Verification items for the finished model (mm, model axes). A direction names the side the tool comes from. Coordinates: 2 decimals unless noted, no trailing zeros. Order: outer loops, then holes, each group sorted by start corner. A loop starts at its lowest first (then second) coordinate and runs counter-clockwise, first axis right, second up. Notation, with made-up numbers: (33, 0.25) -> (63, 0.25) arc R31 ccw to (63, 38.25) -> close; hole circle Ø1 at (-8, 55.5). An arc over 180 degrees is marked (long way). Use CSV: the item, a comma, the result in double quotes. Start each with the question number.
1) Sectioned sample at C-C on z = 0. Record the boundary of the cut face in (x, y).
2) Release check for a two-part mould opening along Z. For faces 1 (the flat face through (0, 6, -30)), 2 (the flat face through (20, 2, -24.207)), 3 (the cylindrical face through (-0.521, 15.966, 28.986)) record: released by +Z, released by -Z, zero draft, split by the parting line, or undercut.
3) Sectioned sample at D-D on y = 12. Record the boundary of the cut face in (x, z).
4) Tool access check on faces 4 (the flat face through (-7, 2, 24)), 5 (the flat face through (0, 6, 30)), 6 (the flat face through (18, 18, -27)). Record the directions out of +Z, -Z, +X, -X, +Y, -Y that give a thin tool (end or side, any length) a straight path to the whole face; none if there is none.
5) Go/stop test with flat-tipped pins: pin 1 (2.5 mm diameter, centred on y = 20.5, z = -22.5, fed in from -X); pin 2 (1.5 mm diameter, centred on y = 9, z = 1.5, fed in from +X); pin 3 (1 mm diameter, centred on x = 18, z = 27.5, fed in from +Y). Record where each tip stops, or that it passes through.
6) Sectioned sample at A-A on y = 5.5. Give the number of separate pieces and of enclosed holes in the cut face, then the cut area to 3 significant figures.
7) Scan lines: line 1 along X through (y, z) = (19.3, -27.5); line 2 along Y through (x, z) = (15.5, -22.5); line 3 along X through (y, z) = (19, 4). Record each from-to range of solid material in increasing order.
8) Sectioned sample at B-B on x = 0. Record the boundary of the cut face in (y, z), then the cut area to 3 significant figures.
from build123d import *

# Parameters (mm, degrees)
CROQUIS2_R                 = 1.5
SALIENTE_EXTRUIR1_DEPTH    = 3
CROQUIS3_W                 = 1.97
CROQUIS3_H                 = 56
SALIENTE_EXTRUIR2_DEPTH    = 20
CROQUIS4_W                 = 4.999751321
CROQUIS4_H                 = 20
SALIENTE_EXTRUIR3_DEPTH    = 5
CROQUIS5_W                 = 5
CROQUIS5_H                 = 20
SALIENTE_EXTRUIR4_DEPTH    = 5
CROQUIS6_R                 = 1
CORTAR_EXTRUIR1_DEPTH      = 5
CROQUIS7_R                 = 1
CORTAR_EXTRUIR2_DEPTH      = 67.738294854
CROQUIS8_R                 = 1
CORTAR_EXTRUIR3_DEPTH      = 67.713573581
CROQUIS9_W                 = 6
CROQUIS9_H                 = 20
CORTAR_EXTRUIR5_DEPTH      = 10
CORTAR_EXTRUIR6_DEPTH      = 76.166481892
CORTAR_EXTRUIR6_DEPTH_BACK = 76.166481892
CROQUIS10_R                = 4


with BuildPart() as part:
    # Croquis2 → Saliente-Extruir1 (new body)
    with BuildSketch(Plane(origin=(0, 0, 0), x_dir=(1, 0, 0), z_dir=(0, 1, 0))):
        with BuildLine():
            Line((-24.919871589, 30), (24.919871589, 30))
            ThreePointArc((24.919871589, 30), (39, 0), (24.919871589, -30))
            Line((24.919871589, -30), (-24.919871589, -30))
            ThreePointArc((-24.919871589, -30), (-39, 0), (-24.919871589, 30))
        make_face()
        with Locations(Location((-24, 26.5, 0), (0, 0, 270))):
            Circle(CROQUIS2_R, mode=Mode.SUBTRACT)
        with Locations(Location((24, 26.5, 0), (0, 0, 90))):
            Circle(CROQUIS2_R, mode=Mode.SUBTRACT)
        with Locations(Location((-24, -26.5, 0), (0, 0, 90))):
            Circle(CROQUIS2_R, mode=Mode.SUBTRACT)
        with Locations(Location((24, -26.5, 0), (0, 0, 270))):
            Circle(CROQUIS2_R, mode=Mode.SUBTRACT)
    extrude(amount=SALIENTE_EXTRUIR1_DEPTH)

    # Croquis3 → Saliente-Extruir2 (add)
    with BuildSketch(Plane(origin=(0, 3, 0), x_dir=(1, 0, 0), z_dir=(0, 1, 0))):
        Polygon((-16, 28), (-16, -28), (-14, -28), (-14, 0), (-14, 28), align=None)
        with Locations((14.985, 0)):
            Rectangle(CROQUIS3_W, CROQUIS3_H)
        Polygon((-16, 28), (-14, 28), (0, 28), (14, 28), (15.97, 28), (15.97, 30), (-16, 30), align=None)
        Polygon((14, -28), (-14, -28), (-16, -28), (-16, -30), (15.97, -30), (15.97, -28), align=None)
    extrude(amount=SALIENTE_EXTRUIR2_DEPTH)

    # Croquis4 → Saliente-Extruir3 (add)
    with BuildSketch(Plane(origin=(15.97, 0, 0), x_dir=(0, 0, -1), z_dir=(1, 0, 0))):
        with Locations((27.50012434, 13)):
            Rectangle(CROQUIS4_W, CROQUIS4_H)
        with Locations((-27.50012434, 13)):
            Rectangle(CROQUIS4_W, CROQUIS4_H)
    extrude(amount=SALIENTE_EXTRUIR3_DEPTH)

    # Croquis5 → Saliente-Extruir4 (add)
    with BuildSketch(Plane.ZY.offset(16)):
        with Locations((-27.5, 13)):
            Rectangle(CROQUIS5_W, CROQUIS5_H)
        with Locations((27.5, 13)):
            Rectangle(CROQUIS5_W, CROQUIS5_H)
    extrude(amount=SALIENTE_EXTRUIR4_DEPTH)

    # Croquis6 → Cortar-Extruir1 (cut)
    with BuildSketch(Plane(origin=(0, 23, 0), x_dir=(1, 0, 0), z_dir=(0, 1, 0))):
        with Locations(Location((18.47, -27.5, 0), (0, 0, 270))):
            Circle(CROQUIS6_R)
        with Locations(Location((18.47, 27.5, 0), (0, 0, 90))):
            Circle(CROQUIS6_R)
        with Locations(Location((-17.474298495, -27.5, 0), (0, 0, 90))):
            Circle(CROQUIS6_R)
        with Locations(Location((-17.474298495, 27.5, 0), (0, 0, 270))):
            Circle(CROQUIS6_R)
    extrude(amount=-CORTAR_EXTRUIR1_DEPTH, mode=Mode.SUBTRACT)

    # Croquis7 → Cortar-Extruir2 (cut, through all)
    with BuildSketch(Plane.ZY.offset(16)):
        with Locations((-22.5, 5.5)):
            Circle(CROQUIS7_R)
        with Locations((22.5, 5.5)):
            Circle(CROQUIS7_R)
    extrude(amount=-CORTAR_EXTRUIR2_DEPTH, mode=Mode.SUBTRACT)

    # Croquis8 → Cortar-Extruir3 (cut, through all)
    with BuildSketch(Plane(origin=(15.97, 0, 0), x_dir=(0, 0, -1), z_dir=(1, 0, 0))):
        with Locations((22.500248679, 20.5)):
            Circle(CROQUIS8_R)
        with Locations((-22.500248679, 20.5)):
            Circle(CROQUIS8_R)
    extrude(amount=-CORTAR_EXTRUIR3_DEPTH, mode=Mode.SUBTRACT)

    # Croquis9 → Cortar-Extruir5 (cut)
    with BuildSketch(Plane(origin=(0, 3, 0), x_dir=(1, 0, 0), z_dir=(0, 1, 0))):
        with BuildLine():
            Line((15.97, 10.29364367), (15.97, 17.915331423))
            ThreePointArc((15.97, 17.915331423), (21.003069429, 11.613400646), (23.664319132, 4))
            Line((23.664319132, 4), (18.574175621, 4))
            ThreePointArc((18.574175621, 4), (17.556409228, 7.264467978), (15.97, 10.29364367))
        make_face()
        with BuildLine():
            Line((15.97, -10.29364367), (15.97, -17.915331423))
            ThreePointArc((15.97, -17.915331423), (21.003069429, -11.613400646), (23.664319132, -4))
            Line((23.664319132, -4), (18.574175621, -4))
            ThreePointArc((18.574175621, -4), (17.556409228, -7.264467978), (15.97, -10.29364367))
        make_face()
        with BuildLine():
            Line((15.97, 24.206592077), (23.875529314, 24.206592077))
            ThreePointArc((23.875529314, 24.206592077), (30.539353975, 14.944827159), (33.763886032, 4))
            Line((33.763886032, 4), (28.722813233, 4))
            ThreePointArc((28.722813233, 4), (24.52424269, 15.47777505), (15.97, 24.206592077))
        make_face()
        with BuildLine():
            Line((15.97, -24.206592077), (23.875529314, -24.206592077))
            ThreePointArc((23.875529314, -24.206592077), (30.539353975, -14.944827159), (33.763886032, -4))
            Line((33.763886032, -4), (28.722813233, -4))
            ThreePointArc((28.722813233, -4), (24.52424269, -15.47777505), (15.97, -24.206592077))
        make_face()
        with BuildLine():
            Line((-15.97, -10.29364367), (-15.97, -17.915331423))
            ThreePointArc((-15.97, -17.915331423), (-21.003069429, -11.613400646), (-23.664319132, -4))
            Line((-23.664319132, -4), (-18.574175621, -4))
            ThreePointArc((-18.574175621, -4), (-17.556409228, -7.264467978), (-15.97, -10.29364367))
        make_face()
        with BuildLine():
            Line((-15.97, 10.29364367), (-15.97, 17.915331423))
            ThreePointArc((-15.97, 17.915331423), (-21.003069429, 11.613400646), (-23.664319132, 4))
            Line((-23.664319132, 4), (-18.574175621, 4))
            ThreePointArc((-18.574175621, 4), (-17.556409228, 7.264467978), (-15.97, 10.29364367))
        make_face()
        with BuildLine():
            Line((-15.97, 24.206592077), (-23.875529314, 24.206592077))
            ThreePointArc((-23.875529314, 24.206592077), (-30.539353975, 14.944827159), (-33.763886032, 4))
            Line((-33.763886032, 4), (-28.722813233, 4))
            ThreePointArc((-28.722813233, 4), (-24.52424269, 15.47777505), (-15.97, 24.206592077))
        make_face()
        with BuildLine():
            Line((-15.97, -24.206592077), (-23.875529314, -24.206592077))
            ThreePointArc((-23.875529314, -24.206592077), (-30.539353975, -14.944827159), (-33.763886032, -4))
            Line((-33.763886032, -4), (-28.722813233, -4))
            ThreePointArc((-28.722813233, -4), (-24.52424269, -15.47777505), (-15.97, -24.206592077))
        make_face()
        with Locations((-7, 14)):
            Rectangle(CROQUIS9_W, CROQUIS9_H)
        with Locations((7, 14)):
            Rectangle(CROQUIS9_W, CROQUIS9_H)
        with Locations((7, -14)):
            Rectangle(CROQUIS9_W, CROQUIS9_H)
        with Locations((-7, -14)):
            Rectangle(CROQUIS9_W, CROQUIS9_H)
    extrude(amount=-CORTAR_EXTRUIR5_DEPTH, mode=Mode.SUBTRACT)

    # Croquis10 → Cortar-Extruir6 (cut, two sides: drawn at the far end of the back side and taken through both)
    with BuildSketch(Plane.XY.offset(30).offset(-CORTAR_EXTRUIR6_DEPTH_BACK)):
        with Locations((0, 12)):
            Circle(CROQUIS10_R)
    extrude(amount=CORTAR_EXTRUIR6_DEPTH + CORTAR_EXTRUIR6_DEPTH_BACK, mode=Mode.SUBTRACT)


solid = part.part
Answers follow:
1,outline,"(-39, 0) -> (39, 0) -> (39, 3) -> (15.97, 3) -> (15.97, 23) -> (14, 23) -> (14, 3) -> (-14, 3) -> (-14, 23) -> (-16, 23) -> (-16, 3) -> (-39, 3) -> close"
2,face 1,"released by -Z"
2,face 2,"undercut"
2,face 3,"zero draft"
3,outline,"(-21, -30) -> (-4, -30) -> (-4, -28) -> (-14, -28) -> (-14, 28) -> (-4, 28) -> (-4, 30) -> (-21, 30) -> (-21, 25) -> (-16, 25) -> (-16, -25) -> (-21, -25) -> close; (4, -30) -> (20.97, -30) -> (20.97, -25) -> (15.97, -25) -> (15.97, 25) -> (20.97, 25) -> (20.97, 30) -> (4, 30) -> (4, 28) -> (14, 28) -> (14, -28) -> (4, -28) -> close"
4,face 4,"+Y, -Y"
4,face 5,"+Z, +X, -X, +Y, -Y"
4,face 6,"+Y"
5,pin 1,"stops at x = -16"
5,pin 2,"stops at x = 15.97"
5,pin 3,"stops at y = 18"
6,separate pieces,"4"
6,enclosed holes,"0"
6,area,"434 mm²"
7,line 1,"x = -21 to -18.47, -16.47 to -14, 14 to 17.47, 19.47 to 20.97"
7,line 2,"y = 0 to 4.5, 6.5 to 19.5, 21.5 to 23"
7,line 3,"x = -16 to -14, 14 to 15.97"
8,outline,"(0, -30) -> (8, -30) -> (8, -28) -> (3, -28) -> (3, 28) -> (8, 28) -> (8, 30) -> (0, 30) -> close; (16, -30) -> (23, -30) -> (23, -28) -> (16, -28) -> close; (16, 28) -> (23, 28) -> (23, 30) -> (16, 30) -> close"
8,area,"228 mm²"
